Work out the finished part from the listing and answer in its coordinate system (mm). A direction names the side the tool comes from. Round coordinates to 2 decimals unless told otherwise and drop trailing zeros. Write each loop counter-clockwise with the first axis right and the second up, starting at its lowest first coordinate (ties: lowest second). Pieces come first, ordered by that corner, then holes.
1. A tool of negligible diameter and unlimited length cuts with its end or side. For faces 4 (the face through (66.25, 2, -6)), 5 (the face through (63.25, 2, -7)), from which of +Z, -Z, +X, -X, +Y, -Y can it reach the whole face along a straight path? Write none if from no direction.
2. Find section B-B (y = 24.5). Write down the section's boundary in (x, z), and give its area (3 significant figures).
3. Find section D-D (x = 50). Write down the section's boundary in (y, z).
4. Find section C-C (z = -1). Write down the section's boundary in (x, y).
5. Straight lines are drawn through the part: probe 1 along X at (y, z) = (7, -5.25); probe 2 along Y at (x, z) = (27.75, 2.15); probe 3 along Y at (x, z) = (62.5, -14). For each, find the intervals that lie inside material, in ascending order.
6. Determine the mould class of faces 1 (the face through (19, 3, 3)), 2 (the face through (28, -35.357, -6)), 3 (the face through (46.454, 2.48, 1.479)) for opening direction Y: pulls with the +Y half, pulls with the -Y half, needs draft (parallel to the pull), parting line crosses it, or undercut.
7. Flat-ended cylindrical pins translate along their axes: pin 1 Ø16 at (x, y) = (27.75, 2.64) entering from -Z; pin 2 Ø6 at (x, y) = (5.35, 2.64) entering from -Z; pin 3 Ø8.5 at (x, y) = (50.15, 2.64) entering from +Z. Find the tip coordinate at first contact, or state that the pin passes through.
8. Find section A-A (x = 5.35). Write down the section's boundary in (y, z), and give its area (3 significant figures).
Autodesk Inventor part; units mm, degrees
ref_plane "YZ Plane" through (0, 0, 0) normal (1, 0, 0) x (0, 1, 0)
ref_plane "XZ Plane" through (0, 0, 0) normal (0, 1, 0) x (-1, 0, 0)
ref_plane "XY Plane" through (0, 0, 0) normal (0, 0, 1) x (1, 0, 0)
sketch "Boceto1" plane through (0, 0, 0) normal (0, 0, 1) x (1, 0, 0)
  arc A0 (-1.75, 0) -> (-0.6468, -1.6261) centre (0, 0) ccw
  line L0 (-1.75, 0) -> (-1.75, 5.2862)
  arc A1 (-0.6468, 6.9123) -> (-1.75, 5.2862) centre (0, 5.2862) ccw
  line L1 (-0.6468, 6.9123) -> (12.6254, 12.1912)
  arc A2 (12.6254, 12.1912) -> (13.6116, 12.956) centre (11.7938, 14.2819) ccw
  arc A3 (41.8884, 12.956) -> (13.6116, 12.956) centre (27.75, 2.6431) ccw
  arc A4 (41.8884, 12.956) -> (42.8746, 12.1912) centre (43.7062, 14.2819) ccw
  line L2 (42.8746, 12.1912) -> (56.1468, 6.9123)
  arc A5 (57.25, 5.2862) -> (56.1468, 6.9123) centre (55.5, 5.2862) ccw
  line L3 (57.25, 5.2862) -> (57.25, 0)
  arc A6 (56.1468, -1.6261) -> (57.25, 0) centre (55.5, 0) ccw
  line L4 (56.1468, -1.6261) -> (42.8746, -6.905)
  arc A7 (42.8746, -6.905) -> (41.8884, -7.6698) centre (43.7062, -8.9957) ccw
  arc A8 (13.6116, -7.6698) -> (41.8884, -7.6698) centre (27.75, 2.6431) ccw
  arc A9 (13.6116, -7.6698) -> (12.6254, -6.905) centre (11.7938, -8.9957) ccw
  line L5 (12.6254, -6.905) -> (-0.6468, -1.6261)
  circle A10 centre (50.15, 2.6431) radius 3.7
  circle A11 centre (5.35, 2.6431) radius 3.7
  arc A12 (44.3063, 7.4106) -> (11.1937, 7.4106) centre (27.75, 2.6431) ccw
  arc A13 (11.1937, 7.4106) -> (11.3578, 5.7658) centre (13.3357, 6.7938) ccw
  arc A14 (11.3578, -0.4796) -> (11.3578, 5.7658) centre (5.35, 2.6431) ccw
  arc A15 (11.3578, -0.4796) -> (11.1937, -2.1244) centre (13.3357, -1.5076) ccw
  arc A16 (11.1937, -2.1244) -> (44.3063, -2.1244) centre (27.75, 2.6431) ccw
  arc A17 (44.3063, -2.1244) -> (44.1422, -0.4796) centre (42.1643, -1.5076) ccw
  arc A18 (44.1422, 5.7658) -> (44.1422, -0.4796) centre (50.15, 2.6431) ccw
  arc A19 (44.1422, 5.7658) -> (44.3063, 7.4106) centre (42.1643, 6.7938) ccw
  line L6 (-6.75, 37.6431) -> (63.25, 37.6431)
  line L7 (63.25, 37.6431) -> (63.25, -32.3569)
  line L8 (63.25, -32.3569) -> (-6.75, -32.3569)
  line L9 (-6.75, -32.3569) -> (-6.75, 37.6431)
  line L10 (-6.75, 2.6431) -> (63.25, 2.6431) construction
  point P0 (-1.75, 2.6431)
  dimension "d0" = 70
  dimension "d1" = 70
  dimension "d16" = 35
extrude "Extrusión1" add sketch "Boceto1" along normal blind 3 contours L0 A1 L1 A2 A3 A4 L2 A5 L3 A6 L4 A7 A8 A9 L5 A0 | A19 A18 A17 A16 A15 A14 A13 A12 | L6 L7 L8 L9
sketch "Boceto2" plane through (0, 0, 0) normal (0, 0, -1) x (-1, 0, 0)
  circle A0 centre (-27.75, 2.6431) radius 5
  line L0 (6.75, -32.3569) -> (-63.25, -32.3569)
  line L1 (6.75, 37.6431) -> (6.75, -32.3569)
  line L2 (-63.25, 37.6431) -> (6.75, 37.6431)
  line L3 (-63.25, -32.3569) -> (-63.25, 37.6431)
  circle A1 centre (-5.35, 2.6431) radius 3.7
  circle A2 centre (-50.15, 2.6431) radius 3.7
  line L4 (-66.25, -35.3569) -> (9.75, -35.3569)
  line L5 (9.75, -35.3569) -> (9.75, 40.6431)
  line L6 (9.75, 40.6431) -> (-66.25, 40.6431)
  line L7 (-66.25, 40.6431) -> (-66.25, -35.3569)
  point P0 (0, 0)
  dimension "d6" = 3
extrude "Extrusión2" cut sketch "Boceto2" against normal through all contours A0
sketch "Boceto4" plane through (0, 0, 0) normal (0, 0, -1) x (-1, 0, 0)
  circle A0 centre (-27.75, 2.6431) radius 5
  line L0 (6.75, -32.3569) -> (-63.25, -32.3569)
  line L1 (6.75, 37.6431) -> (6.75, -32.3569)
  line L2 (-63.25, 37.6431) -> (6.75, 37.6431)
  line L3 (-63.25, -32.3569) -> (-63.25, 37.6431)
  circle A1 centre (-5.35, 2.6431) radius 3.7
  circle A2 centre (-50.15, 2.6431) radius 3.7
  line L4 (9.75, -35.3569) -> (-66.25, -35.3569)
  line L5 (-66.25, -35.3569) -> (-66.25, 40.6431)
  line L6 (-66.25, 40.6431) -> (9.75, 40.6431)
  line L7 (9.75, 40.6431) -> (9.75, -35.3569)
  point P0 (0, 0)
  dimension "d9" = 3
extrude "Extrusión3" add sketch "Boceto4" along normal blind 15 and the other way blind 3 contours L4 L5 L6 L7
properties part number "estructura_sensor_chumacera"
Worked answers:
1. face 4: +Z, -Z, +X, +Y, -Y
1. face 5: -Z
2. outline: (-9.75, -15) - (-6.75, -15) - (-6.75, 0) - (63.25, 0) - (63.25, -15) - (66.25, -15) - (66.25, 3) - (-9.75, 3) - close
2. area: 318 mm2
3. outline: (-35.36, -15) - (-32.36, -15) - (-32.36, 0) - (-1.05, 0) - (-1.05, 3) - (-35.36, 3) - close; (6.34, 0) - (37.64, 0) - (37.64, -15) - (40.64, -15) - (40.64, 3) - (6.34, 3) - close
4. outline: (-9.75, -35.36) - (66.25, -35.36) - (66.25, 40.64) - (-9.75, 40.64) - close; hole (-6.75, -32.36) - (63.25, -32.36) - (63.25, 37.64) - (-6.75, 37.64) - close
5. probe 1: x = -9.75 to -6.75, 63.25 to 66.25
5. probe 2: y = -35.36 to -2.36, 7.64 to 40.64
5. probe 3: y = -35.36 to -32.36, 37.64 to 40.64
6. face 1: needs draft
6. face 2: pulls with the -Y half
6. face 3: undercut
7. pin 1: stops at z = 0
7. pin 2: passes through
7. pin 3: stops at z = 3
8. outline: (-35.36, -15) - (-32.36, -15) - (-32.36, 0) - (-1.06, 0) - (-1.06, 3) - (-35.36, 3) - close; (6.34, 0) - (37.64, 0) - (37.64, -15) - (40.64, -15) - (40.64, 3) - (6.34, 3) - close
8. area: 296 mm2
